```python
from build123d import *

# Parameters (mm, degrees)
SKETCH1_R           = 11.5062
BOSS_EXTRUDE1_DEPTH = 4.7625
BOSS_EXTRUDE2_DEPTH = 3.175
FILLET2_R           = 1.5875


with BuildPart() as part:
    # Sketch1 → Boss-Extrude1 (new body, symmetric)
    with BuildSketch(Plane.XY):
        with BuildLine():
            ThreePointArc((14.639156809, 1.110279863), (-4.45502565, 13.988937769), (-12.585193267, -7.559797873))
            ThreePointArc((-12.585193267, -7.559797873), (4.45502565, -13.988937769), (14.639156809, 1.110279863))
        make_face()
        Circle(SKETCH1_R, mode=Mode.SUBTRACT)
    extrude(amount=BOSS_EXTRUDE1_DEPTH, both=True)

    # Sketch5 → Boss-Extrude2 (add, symmetric)
    with BuildSketch(Plane.XY):
        with BuildLine():
            ThreePointArc((-12.585193267, -7.559797873), (-10.89585042, -11.492870345), (-10.31875, -15.734319794))
            Line((-10.31875, -15.734319794), (-10.31875, -49.389319794))
            Line((-10.31875, -49.389319794), (8.54075, -49.389319794))
            Line((8.54075, -49.389319794), (8.54075, -76.059319794))
            Line((8.54075, -76.059319794), (37.089554297, -67.094446092))
            Line((37.089554297, -67.094446092), (21.666696712, -45.336128971))
            Line((21.666696712, -45.336128971), (37.052935248, -34.429965394))
            Line((37.052935248, -34.429965394), (17.517315641, -6.869430374))
            ThreePointArc((17.517315641, -6.869430374), (15.535368252, -3.075379389), (14.639156809, 1.110279863))
            ThreePointArc((14.639156809, 1.110279863), (4.45502565, -13.988937769), (-12.585193267, -7.559797873))
        make_face()
        with BuildLine():
            ThreePointArc((5.55625, -39.070569794), (0, -44.626819794), (-5.55625, -39.070569794))
            Line((-5.55625, -39.070569794), (-5.55625, -27.958069794))
            ThreePointArc((-5.55625, -27.958069794), (0, -22.401819794), (5.55625, -27.958069794))
            Line((5.55625, -27.958069794), (5.55625, -39.070569794))
        make_face(mode=Mode.SUBTRACT)
        with BuildLine():
            ThreePointArc((27.200344435, -28.7656506), (25.880457031, -36.511728663), (18.134378968, -35.19184126))
            Line((18.134378968, -35.19184126), (11.708188308, -26.125875793))
            ThreePointArc((11.708188308, -26.125875793), (13.028075711, -18.379797729), (20.774153775, -19.699685133))
            Line((20.774153775, -19.699685133), (27.200344435, -28.7656506))
        make_face(mode=Mode.SUBTRACT)
    extrude(amount=BOSS_EXTRUDE2_DEPTH, both=True)

    # Fillet2
    fillet2_edges = [part.edges().sort_by_distance(p)[0] for p in [
        (37.089554297, -67.094446092, 0),
        (21.666696712, -45.336128971, 0),
        (37.052935248, -34.429965394, 0),
        (-10.31875, -49.389319794, 0),
        (8.54075, -49.389319794, 0),
        (8.54075, -76.059319794, 0),
    ]]
    fillet(fillet2_edges, radius=FILLET2_R)


solid = part.part
```
Verification items for the finished model (mm, model axes). A direction names the side the tool comes from. Round coordinates to 2 decimals unless told otherwise and drop trailing zeros. Order: outer loops, then holes, each group sorted by start corner. A loop starts at its lowest first (then second) coordinate and runs counter-clockwise, first axis right, second up. Notation, with made-up numbers: (48.25, 3.5) -> (83.25, 3.5) arc R23 cw to (83.25, 39.5) -> close; hole circle Ø11 at (41, -25.5). An arc over 180 degrees is marked (long way). Put each result on its own line as item: value. Start each with the question number.
(1) Section check B-B (z = 2). State how many separate pieces and enclosed holes the cut face has, then the cut area to 3 significant figures.
(2) Section check A-A (x = 0). Enter the section's corners in (y, z) (1 decimal), then the cut area to 3 significant figures.
(3) Section check C-C (x = 30). Enter the section's corners in (y, z) (3 decimals), then the cut area to 3 significant figures.
(4) Tool access check on faces 1 (the face through (22.64, -71.63, 0.04)), 2 (the face through (29.299, -56.104, 0.044)), 3 (the face through (14.966, -30.722, 0.044)), 4 (the face through (-1, -49.389, 0)). Record the directions out of +Z, -Z, +X, -X, +Y, -Y that give a thin tool (end or side, any length) a straight path to the whole face; none if there is none.
(5) Draft check along X on faces 5 (the face through (5.556, -33, 0)), 6 (the face through (-10.319, -32, 0)), 7 (the face through (12.93, -18.45, 0.04)), 8 (the face through (-9, -8, 4.762)). Enter one of: +X half, -X half, draft (parallel to the pull), parting line (faces both ways), or undercut.
(6) Material ranges on line 1 along Y through (x, z) = (0, 2.3); line 2 along Y through (x, z) = (0, -3.65); line 3 along X through (y, z) = (-24.5, -2.75), recorded low to high.
(7) Depth check by flat-ended pin: pin 1 Ø1.9 at (y, z) = (-67, 0) entering from -X; pin 2 Ø2 at (y, z) = (-31.5, 0.5) entering from +X; pin 3 Ø1.5 at (x, z) = (-8, 3.5) entering from -Y. Enter the tip coordinate at first touch or a pass-through.
Completed:
1. separate pieces: 1
1. enclosed holes: 3
1. area: 1,820 mm2
2. outline: (-49.4, -3.2) -> (-44.6, -3.2) -> (-44.6, 3.2) -> (-49.4, 3.2) -> close; (-22.4, -3.2) -> (-14.7, -3.2) -> (-14.7, -4.8) -> (-11.5, -4.8) -> (-11.5, 4.8) -> (-14.7, 4.8) -> (-14.7, 3.2) -> (-22.4, 3.2) -> close; (11.5, -4.8) -> (14.7, -4.8) -> (14.7, 4.8) -> (11.5, 4.8) -> close
2. area: 140 mm2
3. outline: (-69.321, -3.175) -> (-57.093, -3.175) -> (-57.093, 3.175) -> (-69.321, 3.175) -> close; (-39.429, -3.175) -> (-24.48, -3.175) -> (-24.48, 3.175) -> (-39.429, 3.175) -> close
3. area: 173 mm2
4. face 1: +Z, -Z, +X, -Y
4. face 2: +Z, -Z, +X
4. face 3: +Z, -Z
4. face 4: +Z, -Z, -X, -Y
5. face 5: undercut
5. face 6: -X half
5. face 7: undercut
5. face 8: draft
6. line 1: y = -49.39 to -44.63, -22.4 to -11.51, 11.51 to 14.68
6. line 2: y = -14.68 to -11.51, 11.51 to 14.68
6. line 3: x = -10.32 to -4.35, 4.35 to 10.92, 24.18 to 30.01
7. pin 1: stops at x = 8.54
7. pin 2: stops at x = 35.68
7. pin 3: stops at y = -49.39
